from build123d import *

# Parameters (mm, degrees)
SKETCH1_R           = 3.175
BOSS_EXTRUDE1_DEPTH = 3
SKETCH2_W           = 9
SKETCH2_H           = 10
BOSS_EXTRUDE2_DEPTH = 3
SKETCH3_W           = 30
SKETCH3_H           = 10
BOSS_EXTRUDE3_DEPTH = 3
BOSS_EXTRUDE4_DEPTH = 3
SKETCH6_R           = 3.175
CUT_EXTRUDE1_DEPTH  = 3
SKETCH7_W           = 3
SKETCH7_H           = 8
BOSS_EXTRUDE5_DEPTH = 10


with BuildPart() as part:
    # Sketch1 → Boss-Extrude1 (new body)
    with BuildSketch(Plane.XY):
        with BuildLine():
            Line((0, 0), (25, 0))
            Line((25, 0), (25, 10))
            Line((25, 10), (0, 10))
            ThreePointArc((0, 10), (-5, 5), (0, 0))
        make_face()
        with Locations((0, 5)):
            Circle(SKETCH1_R, mode=Mode.SUBTRACT)
    boss_extrude1 = extrude(amount=BOSS_EXTRUDE1_DEPTH)

    # Sketch2 → Boss-Extrude2 (add)
    with BuildSketch(Plane(origin=(25, 0, 0), x_dir=(0, 0, -1), z_dir=(1, 0, 0))):
        with Locations((1.5, 5)):
            Rectangle(SKETCH2_W, SKETCH2_H)
    boss_extrude2 = extrude(amount=BOSS_EXTRUDE2_DEPTH)

    # Sketch3 → Boss-Extrude3 (add)
    with BuildSketch(Plane(origin=(0, 0, -6), x_dir=(-1, 0, 0), z_dir=(0, 0, -1))):
        with Locations((-40, 5)):
            Rectangle(SKETCH3_W, SKETCH3_H)
    boss_extrude3 = extrude(amount=BOSS_EXTRUDE3_DEPTH)

    # Sketch5 → Boss-Extrude4 (add)
    with BuildSketch(Plane(origin=(0, 0, -9), x_dir=(-1, 0, 0), z_dir=(0, 0, -1))):
        with BuildLine():
            Line((-55, 10), (-55, 0))
            ThreePointArc((-55, 0), (-60, 5), (-55, 10))
        make_face()
    boss_extrude4 = extrude(amount=-BOSS_EXTRUDE4_DEPTH)

    # Sketch6 → Cut-Extrude1 (cut)
    with BuildSketch(Plane(origin=(0, 0, -9), x_dir=(-1, 0, 0), z_dir=(0, 0, -1))):
        with Locations((-55, 5)):
            Circle(SKETCH6_R)
    cut_extrude1 = extrude(amount=-CUT_EXTRUDE1_DEPTH, mode=Mode.SUBTRACT)

    # Sketch7 → Boss-Extrude5 (add)
    with BuildSketch(Plane(origin=(0, 10, 0), x_dir=(1, 0, 0), z_dir=(0, 1, 0))):
        with Locations((26.5, -7)):
            Rectangle(SKETCH7_W, SKETCH7_H)
    boss_extrude5 = extrude(amount=-BOSS_EXTRUDE5_DEPTH)

    # Mirror5: Boss-Extrude1, Boss-Extrude2, Boss-Extrude3, Boss-Extrude4, Cut-Extrude1, Boss-Extrude5 across plane
    add(boss_extrude1.mirror(Plane.XY.offset(5)))
    add(boss_extrude2.mirror(Plane.XY.offset(5)))
    add(boss_extrude3.mirror(Plane.XY.offset(5)))
    add(boss_extrude4.mirror(Plane.XY.offset(5)))
    add(cut_extrude1.mirror(Plane.XY.offset(5)), mode=Mode.SUBTRACT)
    add(boss_extrude5.mirror(Plane.XY.offset(5)))


solid = part.part
The listing builds one solid part. Answer for the finished solid, in the listing's coordinates (mm). A direction names the side the tool comes from. Coordinates: 2 decimals unless noted, no trailing zeros. Loops run counter-clockwise (first coordinate to the right, second up) from the corner with the lowest first, then second, coordinate; pieces in that order, holes last.
1) Find section A-A on y = 5. Give the number of separate pieces and of enclosed holes in the cut face, then the cut area to 3 significant figures.
2) Determine the mould class of faces 5 (the face through (28, 5, 5)), 6 (the face through (25, 5, -4)), 7 (the face through (10, 5, 7)), 8 (the face through (52.07, 3.78, -7.52)) for opening direction X: pulls with the +X half, pulls with the -X half, needs draft (parallel to the pull), parting line crosses it, or undercut.
3) Flat-ended cylindrical pins translate along their axes: pin 1 Ø5 at (x, y) = (0, 5) entering from -Z; pin 2 Ø4.5 at (y, z) = (6, 16.5) entering from -X; pin 3 Ø5 at (x, y) = (7.5, 4) entering from -Z; pin 4 Ø3 at (y, z) = (6.5, 5) entering from +X. Find the tip coordinate at first contact, or state that the pin passes through.
4) Find section D-D on z = -3.75. Write down the section's boundary in (x, y), then the cut area to 3 significant figures.
5) Find section C-C on y = 1. Write down the section's boundary in (x, z).
6) Find section B-B on x = 20. Write down the section's boundary in (y, z).
7) A tool of negligible diameter and unlimited length cuts with its end or side. For faces 1 (the face through (44, 5, -6)), 2 (the face through (-5, 5, 1)), 3 (the face through (10, 5, 0)), 4 (the face through (10, 5, 10)), from which of +Z, -Z, +X, -X, +Y, -Y can it reach the whole face along a straight path? Write none if from no direction.
8) Find the intervals of material crossed by L1, parallel to Z at x = 9.5, y = 4; L2, parallel to Y at x = 55, z = 17.15 (3 decimals); L3, parallel to Z at x = 48, y = 8.5, in increasing order.
Values:
1. separate pieces: 5
1. enclosed holes: 0
1. area: 380 mm2
2. face 5: pulls with the +X half
2. face 6: pulls with the -X half
2. face 7: needs draft
2. face 8: undercut
3. pin 1: passes through
3. pin 2: stops at x = 25
3. pin 3: stops at z = 0
3. pin 4: stops at x = 28
4. outline: (25, 0) - (28, 0) - (28, 10) - (25, 10) - close
4. area: 30.0 mm2
5. outline: (-3, 0) - (25, 0) - (25, -9) - (58, -9) - (58, -6) - (28, -6) - (28, 16) - (58, 16) - (58, 19) - (25, 19) - (25, 10) - (-3, 10) - (-3, 7) - (25, 7) - (25, 3) - (-3, 3) - close
6. outline: (0, 0) - (10, 0) - (10, 3) - (0, 3) - close; (0, 7) - (10, 7) - (10, 10) - (0, 10) - close
7. face 1: +X, +Y, -Y
7. face 2: +Z, -Z, -X
7. face 3: -Z, -X, +Y, -Y
7. face 4: +Z, -X, +Y, -Y
8. L1: z = 0 to 3, 7 to 10
8. L2: y = 0 to 1.825, 8.175 to 10
8. L3: z = -9 to -6, 16 to 19
